from build123d import *
from OCP.BRepFilletAPI import BRepFilletAPI_MakeChamfer

# Parameters (mm, degrees)
SKETCH1_W           = 18
SKETCH1_H           = 20
SKETCH1_R           = 1.45
BOSS_EXTRUDE1_DEPTH = 2
BOSS_EXTRUDE2_DEPTH = 15
BOSS_EXTRUDE4_DEPTH = 1.5
CHAMFER1_SIZE       = 2
CHAMFER1_SIZE2      = 3.571892366
FILLET1_R           = 1.5
FILLET2_R           = 1
FILLET3_R           = 2
FILLET_2_DEPTH      = 1.5


with BuildPart() as part:
    # Sketch1 → Boss-Extrude1 (new body)
    with BuildSketch(Plane(origin=(0, 0, 0), x_dir=(1, 0, 0), z_dir=(0, 1, 0))):
        Rectangle(SKETCH1_W, SKETCH1_H)
        with Locations(Location((3, 7.71, 0), (0, 0, 270))):
            Circle(SKETCH1_R, mode=Mode.SUBTRACT)
        with Locations(Location((3, -7.71, 0), (0, 0, 270))):
            Circle(SKETCH1_R, mode=Mode.SUBTRACT)
    extrude(amount=BOSS_EXTRUDE1_DEPTH)

    # Sketch2 → Boss-Extrude2 (add)
    with BuildSketch(Plane.ZY.offset(9)):
        Polygon((10, 2), (11.5, 2), (17.342742479, 16.7), (31.7, 16.7), (31.7, 14.7), (18.7, 14.7), (12.857257521, 0), (10, 0), align=None)
    extrude(amount=-BOSS_EXTRUDE2_DEPTH)

    # Sketch4 → Boss-Extrude4 (add)
    with BuildSketch(Plane.ZY.offset(9)):
        Polygon((31.7, 16.7), (17.342742479, 16.7), (11.5, 2), (11.5, 10.122171388), (15.306856196, 19.7), (31.7, 19.7), align=None)
    extrude(amount=-BOSS_EXTRUDE4_DEPTH)

    # Chamfer1: one chamfer whose edges measure the first distance from different faces: ONE call of the kernel's chamfer builder (chamfer() names one face for all edges)
    chamfer1_edges_1 = [part.edges().sort_by_distance(p)[0] for p in [
        (-8.25, 19.7, 31.7),
    ]]
    chamfer1_edges_2 = [part.edges().sort_by_distance(p)[0] for p in [
        (-8.25, 19.7, 15.306856196),
    ]]
    chamfer1_side_2 = [part.faces().sort_by_distance(p)[0] for p in [
        (-8.25, 14.911085694, 13.403428098),
    ]]
    chamfer1 = BRepFilletAPI_MakeChamfer(part.part.solid().wrapped)
    for e in chamfer1_edges_1:
        chamfer1.Add(CHAMFER1_SIZE, e.wrapped)
    for e in chamfer1_edges_2:
        chamfer1.Add(CHAMFER1_SIZE, CHAMFER1_SIZE2, e.wrapped, chamfer1_side_2[0].wrapped)  # the first distance lies on this face
    add(Compound.cast(chamfer1.Shape()), mode=Mode.REPLACE)

    # Fillet1
    fillet1_edges = [part.edges().sort_by_distance(p)[0] for p in [
        (-9, 1, -10),
        (9, 1, -10),
        (9, 1, 10),
    ]]
    fillet(fillet1_edges, radius=FILLET1_R)

    # Fillet2
    fillet2_edges = [part.edges().sort_by_distance(p)[0] for p in [
        (6, 15.7, 31.7),
    ]]
    fillet(fillet2_edges, radius=FILLET2_R)

    # Fillet3
    # the kernel refuses this fillet: 2 mm, written as the material it adds along each edge
    with BuildSketch(Plane(origin=(6, 0, 10), x_dir=(0, 0, 1), z_dir=(0, 1, 0))) as fillet3_piece_1_section:
        with BuildLine():
            CenterArc((1.964101615, 2), FILLET3_R, 188.213210702, 81.786789298)
            Line((-0.015385022, 1.714285714), (-0.213333686, 1.685714286))
            ThreePointArc((-0.213333686, 1.685714286), (-0.2, 1.5), (-0.2, 0))
            Line((-0.2, 0), (0, -0.2))
            Line((0, -0.2), (1.964101615, -0.2))
            Line((1.964101615, -0.2), (1.964101615, 0))
        make_face()
    fillet3_piece_1 = extrude(amount=2, mode=Mode.PRIVATE)
    fillet3_piece_1 = split(fillet3_piece_1, bisect_by=Plane(origin=(5.952622656, 0.913834891, 11.068286869), z_dir=(0, -0.3693593568576952, 0.929286643346212)), keep=Keep.TOP, mode=Mode.PRIVATE)
    add(fillet3_piece_1)
    with BuildSketch(Plane(origin=(6, 0, 10), x_dir=(0, 0, 1), z_dir=(0, 1, 0))) as fillet3_piece_2_section:
        with BuildLine():
            CenterArc((1.964101615, 2), FILLET3_R, 188.213210702, 81.786789298)
            Line((-0.015385022, 1.714285714), (-0.213333686, 1.685714286))
            ThreePointArc((-0.213333686, 1.685714286), (-0.2, 1.5), (-0.2, 0))
            Line((-0.2, 0), (0, -0.2))
            Line((0, -0.2), (1.964101615, -0.2))
            Line((1.964101615, -0.2), (1.964101615, 0))
        make_face()
    fillet3_piece_2 = extrude(amount=2, mode=Mode.PRIVATE)
    fillet3_piece_2 = split(fillet3_piece_2, bisect_by=Plane(origin=(6.444718366, 0.756232919, 11.005645527), z_dir=(0, 0.3693593568576952, -0.929286643346212)), keep=Keep.TOP, mode=Mode.PRIVATE)
    add(fillet3_piece_2)
    with BuildSketch(Plane(origin=(6, 0, 10), x_dir=(0, 0, 1), z_dir=(0, 1, 0))) as fillet3_piece_3_section:
        with BuildLine():
            CenterArc((1.964101615, 2), FILLET3_R, 188.213210702, 81.786789298)
            Line((-0.015385022, 1.714285714), (-0.213333686, 1.685714286))
            ThreePointArc((-0.213333686, 1.685714286), (-0.2, 1.5), (-0.2, 0))
            Line((-0.2, 0), (0, -0.2))
            Line((0, -0.2), (1.964101615, -0.2))
            Line((1.964101615, -0.2), (1.964101615, 0))
        make_face()
    fillet3_piece_3 = extrude(amount=6.910254038, mode=Mode.PRIVATE)
    fillet3_piece_3 = split(fillet3_piece_3, bisect_by=Plane(origin=(5.904786251, 2.434661137, 11.672762795), z_dir=(0, -0.3693593568576952, 0.929286643346212)), keep=Keep.TOP, mode=Mode.PRIVATE)
    fillet3_piece_3 = split(fillet3_piece_3, bisect_by=Plane(origin=(5.904786251, 2, 11.804045744), z_dir=(0, 1, 0)), keep=Keep.TOP, mode=Mode.PRIVATE)
    add(fillet3_piece_3)

    # Sketch5 → Fillet 2 (add)
    with BuildSketch(Plane.ZY.offset(9)):
        with BuildLine():
            Line((10, 2), (11.5, 2))
            Line((11.5, 2), (11.5, 3.5))
            ThreePointArc((11.5, 3.5), (11.060660172, 2.439339828), (10, 2))
        make_face()
    extrude(amount=-FILLET_2_DEPTH)


solid = part.part
Build history of the part. All positions in model axes, mm. A direction names the side the tool comes from. Coordinates: 2 decimals unless noted, no trailing zeros. Order: outer loops, then holes, each group sorted by start corner. A loop starts at its lowest first (then second) coordinate and runs counter-clockwise, first axis right, second up. Notation, with made-up numbers: (29.25, 45) - (46.25, 45) arc R15 cw to (46.25, 69) - close; hole circle Ø10 at (-9.75, 77.5). An arc over 180 degrees is marked (long way). Write item = value, one per line. Start each with the question number.
1) Saw through at C-C on x = -0.25. Write the cut outline in (y, z), then the cut area to 3 significant figures.
2) Saw through at D-D on y = 15.5. Write the cut outline in (x, z), then the cut area to 3 significant figures.
3) Saw through at A-A on x = 3. Write the cut outline in (y, z).
4) Saw through at B-B on z = -7.71. Write the cut outline in (x, y).
5) Wall check: line 1 along X through (y, z) = (0.4, 7.71); line 2 along Y through (x, z) = (-0.75, 3.5); line 3 along Y through (x, z) = (5.5, 24.5). Give the ranges that are in metal, low to high. Write a range as from..to.
6) 3-axis set-ups, long thin cutter, end or side, ignore diameter. For faces 1 (the face through (8.55, 1.01, -9.57)), 2 (the face through (-2, 14.7, 25)), 3 (the face through (-1, 16.7, 24)): which of +Z, -Z, +X, -X, +Y, -Y reach the whole face in a straight line?
7) Flat gauge pins, fed straight in: pin 1 Ø1 at (x, y) = (-7, 12) entering from +Z; pin 2 Ø2 at (x, y) = (3, 7.5) entering from +Z; pin 3 Ø4.5 at (x, z) = (3, -7.71) entering from +Y; pin 4 Ø8 at (y, z) = (8, 0.5) entering from +X. Where does each tip first touch, or does it go through?
From the geometry:
q1.outline = (0, -10) - (2, -10) - (2, 11.5) - (16.7, 17.34) - (16.7, 31.7) - (14.7, 31.7) - (14.7, 18.7) - (0, 12.86) - close
q1.area = 103 mm^2
q2.outline = (-9, 13.64) - (-7.5, 13.64) - (-7.5, 16.87) - (6, 16.87) - (6, 30.7) arc R1 ccw to (5, 31.7) - (-9, 31.7) - close
q2.area = 227 mm^2
q3.outline = (0, -10) - (2, -10) - (2, -9.16) - (0, -9.16) - close; (0, -6.26) - (2, -6.26) - (2, 6.26) - (0, 6.26) - close; (0, 9.16) - (2, 9.16) - (2, 11.5) - (16.7, 17.34) - (16.7, 31.7) - (14.7, 31.7) - (14.7, 18.7) - (0, 12.86) - close
q4.outline = (-9, 0) - (1.55, 0) - (1.55, 2) - (-9, 2) - close; (4.45, 0) - (9, 0) - (9, 2) - (4.45, 2) - close
q5.line_1 = -9..1.55, 4.45..9
q5.line_2 = 0..2
q5.line_3 = 14.7..16.7
q6.face_1 = -Z, +X, +Y, -Y
q6.face_2 = +Z, +X, -X, -Y
q6.face_3 = +Z, -Z, +X, +Y
q7.pin_1 = 17.83
q7.pin_2 = 16.24
q7.pin_3 = 2
q7.pin_4 = through
